Read the model definition and answer for the solid it produces. Units are mm, in the model's axes. A direction names the side the tool comes from. Coordinates: 2 decimals unless noted, no trailing zeros. Order: outer loops, then holes, each group sorted by start corner. A loop starts at its lowest first (then second) coordinate and runs counter-clockwise, first axis right, second up.
```python
from build123d import *

# Parameters (mm, degrees)
CROQUIS1_W              = 52
CROQUIS1_H              = 12
CROQUIS1_W_2            = 12.2
CROQUIS1_H_2            = 3.4
SALIENTE_EXTRUIR1_DEPTH = 6
CROQUIS2_R              = 4.15
CORTAR_EXTRUIR1_DEPTH   = 9
CROQUIS3_R              = 1.6
CORTAR_EXTRUIR2_DEPTH   = 30


with BuildPart() as part:
    # Croquis1 → Saliente-Extruir1 (new, symmetric)
    with BuildSketch(Plane.XY):
        Rectangle(CROQUIS1_W, CROQUIS1_H)
        with Locations((13.9, 0)):
            Rectangle(CROQUIS1_W_2, CROQUIS1_H_2, mode=Mode.SUBTRACT)
        with Locations((-13.9, 0)):
            Rectangle(CROQUIS1_W_2, CROQUIS1_H_2, mode=Mode.SUBTRACT)
    extrude(amount=SALIENTE_EXTRUIR1_DEPTH, both=True)

    # Croquis2 → Cortar-Extruir1 (cut)
    with BuildSketch(Plane(origin=(0, 0, -6), x_dir=(-1, 0, 0), z_dir=(0, 0, -1))):
        Circle(CROQUIS2_R)
    extrude(amount=-CORTAR_EXTRUIR1_DEPTH, mode=Mode.SUBTRACT)

    # Croquis3 → Cortar-Extruir2 (cut)
    with BuildSketch(Plane(origin=(0, 6, 0), x_dir=(1, 0, 0), z_dir=(0, 1, 0))):
        with Locations(Location((-13, 0, 0), (0, 0, 180))):
            Circle(CROQUIS3_R)
        with Locations(Location((13, 0, 0), (0, 0, 180))):
            Circle(CROQUIS3_R)
    extrude(amount=-CORTAR_EXTRUIR2_DEPTH, mode=Mode.SUBTRACT)


solid = part.part
```
1) Straight lines are drawn through the part: line 1 (X direction, y = -0.25, z = -3); line 2 (X direction, y = -1, z = 3.25); line 3 (Z direction, x = 13, y = 4.6). For each, find the intervals that lie inside material, in ascending order.
A:
line 1: x = -26 to -20, -7.8 to -4.14, 4.14 to 7.8, 20 to 26
line 2: x = -26 to -20, -7.8 to 7.8, 20 to 26
line 3: z = -6 to -1.6, 1.6 to 6
2) A cutting plane is placed at B-B, the plane x = -10. Determine the outline of the cut face in (y, z).
A:
outline: (-6, -6) - (-1.7, -6) - (-1.7, 6) - (-6, 6) - close; (1.7, -6) - (6, -6) - (6, 6) - (1.7, 6) - close
3) Determine the mould class of faces 4 (the flat face through (-7.8, 0, 0)), 5 (the cylindrical face through (14.6, 3.88, 0.07)), 6 (the flat face through (0, 6, 0)) for opening direction Y: pulls with the +Y half, pulls with the -Y half, needs draft (parallel to the pull), parting line crosses it, or undercut.
A:
face 4: undercut
face 5: needs draft
face 6: pulls with the +Y half
4) A cutting plane is placed at D-D, the plane z = -3.75. Determine the outline of the cut face in (x, y), and give its area (3 significant figures).
A:
outline: (-26, -6) - (26, -6) - (26, 6) - (-26, 6) - close; hole (-20, -1.7) - (-7.8, -1.7) - (-7.8, 1.7) - (-20, 1.7) - close; hole circle Ø8.3 at (0, 0); hole (7.8, -1.7) - (20, -1.7) - (20, 1.7) - (7.8, 1.7) - close
area: 487 mm2
5) A cutting plane is placed at C-C, the plane y = 0. Determine the outline of the cut face in (x, z), and give its area (4 significant figures).
A:
outline: (-26, -6) - (-20, -6) - (-20, 6) - (-26, 6) - close; (-7.8, -6) - (-4.15, -6) - (-4.15, 3) - (4.15, 3) - (4.15, -6) - (7.8, -6) - (7.8, 6) - (-7.8, 6) - close; (20, -6) - (26, -6) - (26, 6) - (20, 6) - close
area: 256.5 mm2
6) A cutting plane is placed at A-A, the plane z = 0. State how many separate pieces and enclosed holes the cut face has, and give its area (3 significant figures).
A:
separate pieces: 3
enclosed holes: 1
area: 432 mm2
7) Which of the six approach directions +Z, -Z, +X, -X, +Y, -Y give full straight-line access (tool end or side, diameter ignored) to faces 1 (the flat face through (0, 0, 3)), 2 (the flat face through (15, -1.7, 0)), 3 (the flat face through (26, 0, 0))?
A:
face 1: -Z
face 2: +Z, -Z
face 3: +Z, -Z, +X, +Y, -Y
